```python
from build123d import *

# Parameters (mm, degrees)
SKETCH1_W           = 76.2
SKETCH1_H           = 38.1
BOSS_EXTRUDE1_DEPTH = 25.4
SKETCH2_W           = 31.75
SKETCH2_H           = 19.05
CUT_EXTRUDE1_DEPTH  = 127
SKETCH3_R           = 3.175
CUT_EXTRUDE2_DEPTH  = 3.175
SKETCH4_R           = 3.175
CUT_EXTRUDE4_DEPTH  = 3.175
SKETCH3_5_R         = 3.175
CUT_EXTRUDE5_DEPTH  = 3.175


with BuildPart() as part:
    # Sketch1 → Boss-Extrude1 (new body)
    with BuildSketch(Plane(origin=(0, 0, 0), x_dir=(1, 0, 0), z_dir=(0, 1, 0))):
        Rectangle(SKETCH1_W, SKETCH1_H)
    extrude(amount=BOSS_EXTRUDE1_DEPTH)

    # Sketch2 → Cut-Extrude1 (cut)
    with BuildSketch(Plane(origin=(38.1, 0, 0), x_dir=(0, 0, -1), z_dir=(1, 0, 0))):
        with Locations((0, 12.7)):
            Rectangle(SKETCH2_W, SKETCH2_H)
    extrude(amount=-CUT_EXTRUDE1_DEPTH, mode=Mode.SUBTRACT)

    # Sketch3 → Cut-Extrude2 (cut)
    with BuildSketch(Plane(origin=(0, 25.4, 0), x_dir=(1, 0, 0), z_dir=(0, 1, 0))):
        with Locations(Location((-25.4, 0, 0), (0, 0, 270))):
            Circle(SKETCH3_R)
        with Locations(Location((0, 0, 0), (0, 0, 270))):
            Circle(SKETCH3_R)
    cut_extrude2 = extrude(amount=-CUT_EXTRUDE2_DEPTH, mode=Mode.SUBTRACT)

    # Mirror1: Cut-Extrude2 across plane
    add(cut_extrude2.mirror(Plane.ZX.offset(12.7)), mode=Mode.SUBTRACT)

    # Sketch4 → Cut-Extrude4 (cut)
    with BuildSketch(Plane.XY.offset(19.05)):
        with Locations((-12.7, 12.7)):
            Circle(SKETCH4_R)
        with Locations((12.7, 12.7)):
            Circle(SKETCH4_R)
    cut_extrude4 = extrude(amount=-CUT_EXTRUDE4_DEPTH, mode=Mode.SUBTRACT)

    # Mirror3: Cut-Extrude4 across plane
    add(cut_extrude4.mirror(Plane.XY), mode=Mode.SUBTRACT)

    # Sketch3_5 → Cut-Extrude5 (cut)
    with BuildSketch(Plane(origin=(0, 25.4, 0), x_dir=(1, 0, 0), z_dir=(0, 1, 0))):
        with Locations(Location((25.4, 0, 0), (0, 0, 270))):
            Circle(SKETCH3_5_R)
    extrude(amount=-CUT_EXTRUDE5_DEPTH, mode=Mode.SUBTRACT)


solid = part.part
```
Check sheet for the modelled part. Datum: model origin and axes. Units: mm. A direction names the side the tool comes from. Coordinates: 2 decimals unless noted, no trailing zeros. Write each loop counter-clockwise with the first axis right and the second up, starting at its lowest first coordinate (ties: lowest second). Pieces come first, ordered by that corner, then holes. Notation, with made-up numbers: (33.25, -40) - (45.25, -40) arc R32 cw to (45.25, -4) - close; hole circle Ø1 at (30.25, -20). An arc over 180 degrees is marked (long way). One line per question, with ' | ' between items.
Item 1: Thickness scan on line 1 (X direction, y = 24.5, z = 0) (3 decimals); line 2 (Y direction, x = -28, z = 8.5) (3 decimals); line 3 (Z direction, x = -6, y = 16) (3 decimals). Record the ranges inside material, lowest first. Write a range as [from, to].
Determined:
line 1: x = [-38.1, -28.575], [-22.225, -3.175], [3.175, 22.225], [28.575, 38.1] | line 2: y = [0, 3.175], [22.225, 25.4] | line 3: z = [-19.05, -15.875], [15.875, 19.05]
Item 2: Sectioned sample at D-D on y = 4.75. Record the boundary of the cut face in (x, z) (3 decimals).
Determined:
outline: (-38.1, -19.05) - (38.1, -19.05) - (38.1, -15.875) - (-38.1, -15.875) - close; (-38.1, 15.875) - (38.1, 15.875) - (38.1, 19.05) - (-38.1, 19.05) - close
Item 3: Access from +Z, -Z, +X, -X, +Y, -Y to the whole of each face (thin tool, end or side, straight path). Record for faces 1 (the face through (-11.2, 9.9, 17.5)), 2 (the face through (28.55, 23.83, -0.41)), 3 (the face through (1, 13, -15.875)).
Determined:
face 1: +Z, -Z | face 2: +Y | face 3: +X, -X
Item 4: Mould release check, pull along X, two halves, no side actions. Record for faces 4 (the face through (-22.25, 1.57, -0.41)), 5 (the face through (1, 13, 15.875)), 6 (the face through (38.1, 24, 0)): pulls with the +X half, pulls with the -X half, needs draft (parallel to the pull), parting line crosses it, or undercut.
Determined:
face 4: undercut | face 5: needs draft | face 6: pulls with the +X half
Item 5: Sectioned sample at A-A on y = 12.7. Record the boundary of the cut face in (x, z) (3 decimals), plus the area to 3 significant figures.
Determined:
outline: (-38.1, -19.05) - (-15.875, -19.05) - (-15.875, -15.875) - (-38.1, -15.875) - close; (-38.1, 15.875) - (-15.875, 15.875) - (-15.875, 19.05) - (-38.1, 19.05) - close; (-9.525, -19.05) - (9.525, -19.05) - (9.525, -15.875) - (-9.525, -15.875) - close; (-9.525, 15.875) - (9.525, 15.875) - (9.525, 19.05) - (-9.525, 19.05) - close; (15.875, -19.05) - (38.1, -19.05) - (38.1, -15.875) - (15.875, -15.875) - close; (15.875, 15.875) - (38.1, 15.875) - (38.1, 19.05) - (15.875, 19.05) - close | area: 403 mm2
Item 6: Sectioned sample at C-C on z = -8. Record the boundary of the cut face in (x, y) (3 decimals), plus the area to 3 significant figures.
Determined:
outline: (-38.1, 0) - (38.1, 0) - (38.1, 3.175) - (-38.1, 3.175) - close; (-38.1, 22.225) - (38.1, 22.225) - (38.1, 25.4) - (-38.1, 25.4) - close | area: 484 mm2
Item 7: Sectioned sample at B-B on x = 0. Record the boundary of the cut face in (y, z) (3 decimals), plus the area to 3 significant figures.
Determined:
outline: (0, -19.05) - (25.4, -19.05) - (25.4, -3.175) - (22.225, -3.175) - (22.225, -15.875) - (3.175, -15.875) - (3.175, -3.175) - (0, -3.175) - close; (0, 3.175) - (3.175, 3.175) - (3.175, 15.875) - (22.225, 15.875) - (22.225, 3.175) - (25.4, 3.175) - (25.4, 19.05) - (0, 19.05) - close | area: 323 mm2
